```python
from build123d import *

# Parameters (mm, degrees)
EXTRUDE1_DEPTH     = 16
FILLET1_R          = 2.5
SKETCH2_R          = 4
CUT_EXTRUDE1_DEPTH = 33
SKETCH3_R          = 4
CUT_EXTRUDE3_DEPTH = 33
SKETCH3_3_R        = 1.85
CUT_EXTRUDE4_DEPTH = 33
SKETCH2_4_R        = 1.85
CUT_EXTRUDE2_DEPTH = 33
CIRPATTERN1_COUNT  = 8
CIRPATTERN3_COUNT  = 8


with BuildPart() as part:
    # Sketch1 → Extrude1 (new body, symmetric)
    with BuildSketch(Plane.XY):
        with BuildLine():
            Line((-13.5, 0), (13.5, 0))
            ThreePointArc((13.5, 0), (15.267766953, 0.732233047), (16, 2.5))
            Line((16, 2.5), (16, 32))
            Line((16, 32), (14, 32))
            Line((14, 32), (14, 2.5))
            ThreePointArc((14, 2.5), (13.853553391, 2.146446609), (13.5, 2))
            Line((13.5, 2), (-13.5, 2))
            ThreePointArc((-13.5, 2), (-13.853553391, 2.146446609), (-14, 2.5))
            Line((-14, 2.5), (-14, 32))
            Line((-14, 32), (-16, 32))
            Line((-16, 32), (-16, 2.5))
            ThreePointArc((-16, 2.5), (-15.267766953, 0.732233047), (-13.5, 0))
        make_face()
    extrude(amount=EXTRUDE1_DEPTH, both=True)

    # Fillet1
    fillet1_edges = [part.edges().sort_by_distance(p)[0] for p in [
        (-15, 32, -16),
        (-15, 32, 16),
        (15, 32, -16),
        (15, 32, 16),
    ]]
    fillet(fillet1_edges, radius=FILLET1_R)

    # Sketch2 → Cut-Extrude1 (cut, through all)
    with BuildSketch(Plane.XZ):
        Circle(SKETCH2_R)
    extrude(amount=-CUT_EXTRUDE1_DEPTH, mode=Mode.SUBTRACT)

    # Sketch3 → Cut-Extrude3 (cut, through all)
    with BuildSketch(Plane.ZY.offset(16)):
        with Locations((0, 16)):
            Circle(SKETCH3_R)
    extrude(amount=-CUT_EXTRUDE3_DEPTH, mode=Mode.SUBTRACT)

    # Sketch3<3> → Cut-Extrude4 (cut, through all)
    with BuildSketch(Plane.ZY.offset(16)):
        with Locations((0, 8)):
            Circle(SKETCH3_3_R)
    cut_extrude4 = extrude(amount=-CUT_EXTRUDE4_DEPTH, mode=Mode.SUBTRACT)

    # Sketch2<4> → Cut-Extrude2 (cut, through all)
    with BuildSketch(Plane.XZ):
        with Locations((8, 0)):
            Circle(SKETCH2_4_R)
    cut_extrude2 = extrude(amount=-CUT_EXTRUDE2_DEPTH, mode=Mode.SUBTRACT)

    # CirPattern1: Cut-Extrude2 ×8 about axis
    cirpattern1_axis = Axis((0, 0, 0), (0, 1, 0))
    for i in range(1, CIRPATTERN1_COUNT):
        add(cut_extrude2.rotate(cirpattern1_axis, i * 360 / CIRPATTERN1_COUNT), mode=Mode.SUBTRACT)

    # CirPattern3: Cut-Extrude4 ×8 about axis
    cirpattern3_axis = Axis((0, 16, 0), (1, 0, 0))
    for i in range(1, CIRPATTERN3_COUNT):
        add(cut_extrude4.rotate(cirpattern3_axis, i * 360 / CIRPATTERN3_COUNT), mode=Mode.SUBTRACT)


solid = part.part
```
Could you check a few things on this model? Use its own coordinates, in mm. A direction names the side the tool comes from. Round coordinates to 2 decimals unless told otherwise and drop trailing zeros. Order: outer loops, then holes, each group sorted by start corner. A loop starts at its lowest first (then second) coordinate and runs counter-clockwise, first axis right, second up. Notation, with made-up numbers: (3.5, 74) -> (14.5, 74) arc R23 ccw to (14.5, 85) -> close; hole circle Ø9 at (-3, 57). An arc over 180 degrees is marked (long way). One line per question, with ' | ' between items.
Q1. If we section it at D-D on z = -8: Write out the boundary of the cut face in (x, y), plus the area to 3 significant figures.
Computed values:
outline: (-16, 2.5) arc R2.5 ccw to (-13.5, 0) -> (-1.85, 0) -> (-1.85, 2) -> (-13.5, 2) arc R0.5 cw to (-14, 2.5) -> (-14, 14.15) -> (-16, 14.15) -> close; (-16, 17.85) -> (-14, 17.85) -> (-14, 32) -> (-16, 32) -> close; (1.85, 0) -> (13.5, 0) arc R2.5 ccw to (16, 2.5) -> (16, 14.15) -> (14, 14.15) -> (14, 2.5) arc R0.5 cw to (13.5, 2) -> (1.85, 2) -> close; (14, 17.85) -> (16, 17.85) -> (16, 32) -> (14, 32) -> close | area: 159 mm²
Q2. If we section it at B-B on y = 16: Give the number of separate pieces and of enclosed holes in the cut face, plus the area to 3 significant figures.
Computed values:
separate pieces: 8 | enclosed holes: 0 | area: 66.4 mm²
Q3. If I drill on line 1 (X direction, y = 5, z = -11); line 2 (Y direction, x = -10, z = -7.5); line 3 (X direction, y = 1, z = -8), over which ranges is the centre line in solid material (lowest first)? Write a range as from..to.
Computed values:
line 1: -16..-14, 14..16 | line 2: 0..2 | line 3: -15.5..-1.85, 1.85..15.5
Q4. I'm going to push flat-ended pins straight in: pin 1 (12 mm diameter, centred on x = 12.5, y = 7.5, fed in from -Z); pin 2 (6 mm diameter, centred on x = 0, z = -8, fed in from +Y); pin 3 (5 mm diameter, centred on y = 16, z = 0, fed in from +X). Where does each tip first touch, or does it pass through?
Computed values:
pin 1: z = -16 | pin 2: y = 2 | pin 3: through
Q5. Which directions (+Z, -Z, +X, -X, +Y, -Y) give clear straight access to the entire face, cutting with the end or side of a thin tool? Please do faces 1 (the face through (3, 0, 4)), 2 (the face through (14, 21, 0)).
Computed values:
face 1: +Z, -Z, +X, -X, -Y | face 2: +Z, -Z, +Y
Q6. If we section it at A-A on x = 8: Write out the boundary of the cut face in (y, z).
Computed values:
outline: (0, -16) -> (2, -16) -> (2, -1.85) -> (0, -1.85) -> close; (0, 1.85) -> (2, 1.85) -> (2, 16) -> (0, 16) -> close
Q7. If we section it at C-C on y = 8: Write out the boundary of the cut face in (x, z), plus the area to 3 significant figures.
Computed values:
outline: (-16, -16) -> (-14, -16) -> (-14, -1.85) -> (-16, -1.85) -> close; (-16, 1.85) -> (-14, 1.85) -> (-14, 16) -> (-16, 16) -> close; (14, -16) -> (16, -16) -> (16, -1.85) -> (14, -1.85) -> close; (14, 1.85) -> (16, 1.85) -> (16, 16) -> (14, 16) -> close | area: 113 mm²
Q8. We'd pull the mould along X, two halves only. Please class faces 3 (the face through (14.99, 17.71, 8.71)), 4 (the face through (-3, 2, 4)), 5 (the face through (-0.08, 0.99, 6.15)), 6 (the face through (15.248, 0.713, 0.224)): released by +X, released by -X, zero draft, split by the parting line, or undercut.
Computed values:
face 3: zero draft | face 4: undercut | face 5: undercut | face 6: released by +X
